For this review, use the dimensioned drawing (mm, ordinates from the lowest corner) and the shaded views. A direction names the side the tool comes from. Coordinates: 2 decimals unless noted, no trailing zeros. Write each loop counter-clockwise with the first axis right and the second up, starting at its lowest first coordinate (ties: lowest second). Pieces come first, ordered by that corner, then holes. Notation, with made-up numbers: (-37.75, 21.5) - (5.25, 21.5) arc R21 cw to (5.25, 35.5) - close; hole circle Ø2 at (3.25, -17.5). An arc over 180 degrees is marked (long way). Use one line per item in the form item = value. Start each with the question number.
1) For L1, parallel to Y at x = 9.5, z = 3.75; L2, parallel to X at y = 11.5, z = 5.25; L3, parallel to X at y = 2.5, z = 3.75, list the stretches that pass through material, from the lowest coordinate up. Write a range as from..to.
2) We need section C-C (y = 18.5). Give the boundary of the cut face in (x, z).
3) We need section A-A (x = 3.25). Give the boundary of the cut face in (y, z), plus the area to 3 significant figures.
4) We need section B-B (z = 5.75). Give the boundary of the cut face in (x, y) (3 decimals), plus the area to 3 significant figures.
5) Insertion check: P1, Ø3, axis at y = 11.5, z = 4, coming from the +X side; P2, Ø1.9, axis at x = 12, z = 3.5, coming from the -Y side. Each pin has a flat end and moves straight along its axis. Give the tip position at first contact, or say it passes through.
6) Tool access review of the marked faces 4 and 5: name each direction out of +Z, -Z, +X, -X, +Y, -Y from which nothing blocks a thin tool from reaching the whole face with its end or side.
7) We need section D-D (z = 2.75). Give the boundary of the cut face in (x, y) (3 decimals).
8) Mouldability with a two-part tool opening along X and no side actions: class the marked faces 1, 2 and 3 as pulls with the +X half, pulls with the -X half, needs draft (parallel to the pull), parting line crosses it, or undercut.
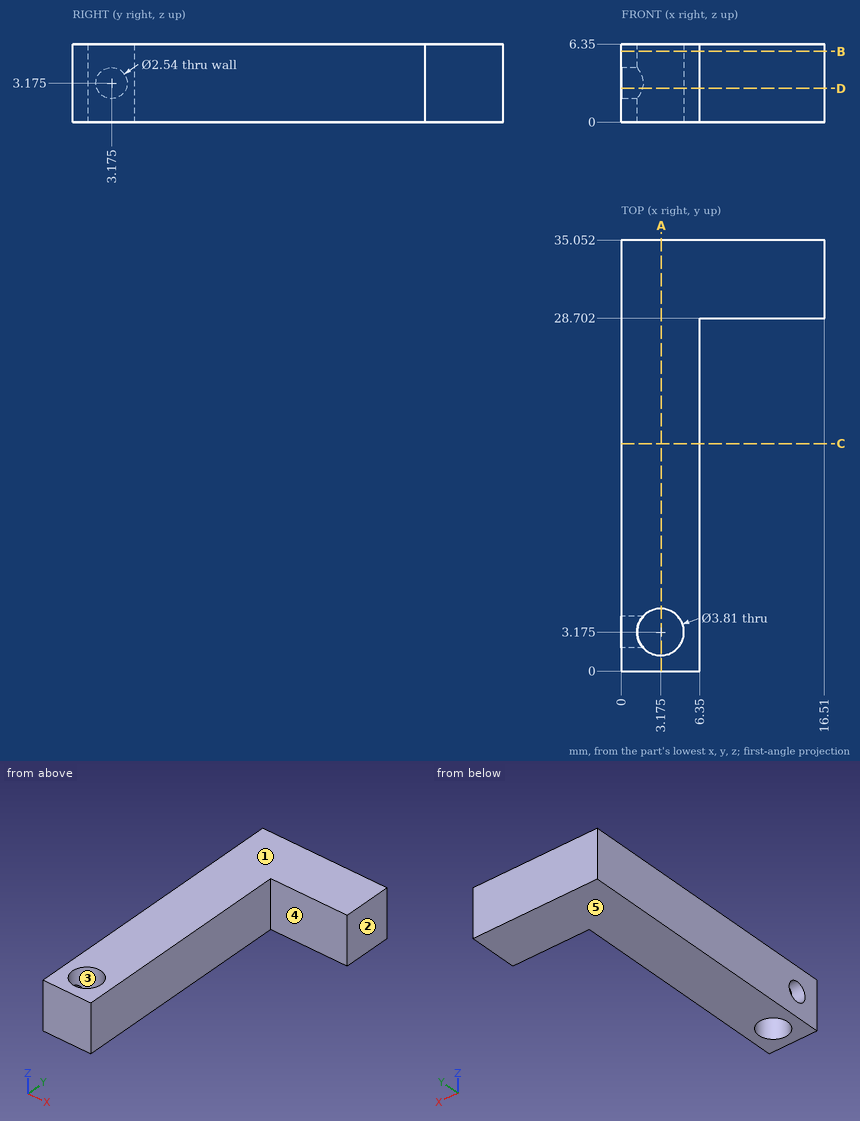
Determined:
q1.L1 = 28.7..35.05
q1.L2 = 0..6.35
q1.L3 = 4.96..6.35
q2.outline = (0, 0) - (6.35, 0) - (6.35, 6.35) - (0, 6.35) - close
q3.outline = (0, 0) - (1.27, 0) - (1.27, 6.35) - (0, 6.35) - close; (5.08, 0) - (35.05, 0) - (35.05, 6.35) - (5.08, 6.35) - close
q3.area = 198 mm²
q4.outline = (0, 0) - (6.35, 0) - (6.35, 28.702) - (16.51, 28.702) - (16.51, 35.052) - (0, 35.052) - close; hole circle Ø3.81 at (3.175, 3.175)
q4.area = 276 mm²
q5.P1 = 6.35
q5.P2 = 28.7
q6.face_4 = +Z, -Z, +X, -Y
q6.face_5 = -Z, +X, -X, +Y, -Y
q7.outline = (0, 0) - (6.35, 0) - (6.35, 28.702) - (16.51, 28.702) - (16.51, 35.052) - (0, 35.052) - (0, 4.372) - (1.693, 4.372) arc R1.905 cw (long way) to (1.693, 1.978) - (0, 1.978) - close
q8.face_1 = needs draft
q8.face_2 = pulls with the +X half
q8.face_3 = undercut
